```python
from build123d import *

# Parameters (mm, degrees)
F0_R      = 1.625
F1_DEPTH  = 8
F2_R      = 2.5
F2_R_2    = 1.625
F3_DEPTH  = 2
F4_R      = 3
F7_R      = 1.125
F8_DEPTH  = 16
F9_R      = 1.125
F10_DEPTH = 4.5
F11_R     = 1.125
F12_DEPTH = 6


with BuildPart() as f1:
    # F0 (on Right) → F1 (new body)
    with BuildSketch(Plane.YZ):
        with BuildLine():
            Line((0, -10), (0, 10))
            Line((0, 10), (-50, 10))
            ThreePointArc((-50, 10), (-60, 0), (-50, -10))
            Line((-50, -10), (0, -10))
        make_face()
        with Locations((-50, 0)):
            Circle(F0_R, mode=Mode.SUBTRACT)
    extrude(amount=F1_DEPTH)

    # F2 (on face) → F3 (join)
    with BuildSketch(Plane.YZ.offset(8)):
        with Locations((-50, 0)):
            Circle(F2_R)
        with Locations((-50, 0)):
            Circle(F2_R_2, mode=Mode.SUBTRACT)
    extrude(amount=F3_DEPTH)

    # F4
    f4_edges = [f1.edges().sort_by_distance(p)[0] for p in [
        (8, -25, 10),
    ]]
    fillet(f4_edges, radius=F4_R)

    # F5: F1 across plane


with BuildPart() as f1_1:
    add(f1.part)
    add(f1.part.mirror(Plane.YZ))

    # F6: F1 across plane


with BuildPart() as f1_2:
    add(f1_1.part)
    add(f1_1.part.mirror(Plane.XZ))

    # F7 (on face) → F8 (cut, through all)
    with BuildSketch(Plane.YZ.offset(8)):
        Polygon((15.6563942954, -6.5), (38.6563942954, -6.5), (38.6563942954, -2.5), (40.1563942954, -2.5), (40.1563942954, 2.5), (38.6563942954, 2.5), (38.6563942954, 6.5), (15.6563942954, 6.5), (15.6563942954, 2.5), (14.1563942954, 2.5), (14.1563942954, -2.5), (15.6563942954, -2.5), align=None)
        with Locations((12.6563942954, 0)):
            Circle(F7_R)
        with Locations((41.6563942954, 0)):
            Circle(F7_R)
    extrude(amount=-F8_DEPTH, mode=Mode.SUBTRACT)

    # F9 (on face) → F10 (cut)
    with BuildSketch(Plane.YZ.offset(8)):
        Polygon((15.6563942954, 6.5), (10.6563942954, 6.5), (10.6563942954, -6.5), (15.6563942954, -6.5), (15.6563942954, -2.5), (14.1563942954, -2.5), (14.1563942954, 2.5), (15.6563942954, 2.5), align=None)
        with Locations((12.6563942954, 0)):
            Circle(F9_R, mode=Mode.SUBTRACT)
        Polygon((43.6563942954, 6.5), (38.6563942954, 6.5), (38.6563942954, 2.5), (40.1563942954, 2.5), (40.1563942954, -2.5), (38.6563942954, -2.5), (38.6563942954, -6.5), (43.6563942954, -6.5), align=None)
        with Locations((41.6563942954, 0)):
            Circle(F9_R, mode=Mode.SUBTRACT)
    extrude(amount=-F10_DEPTH, mode=Mode.SUBTRACT)

    # F11 (on face) → F12 (cut)
    with BuildSketch(Plane(origin=(-8, 0, 0), x_dir=(0, -1, 0), z_dir=(-1, 0, 0))):
        Polygon((-43.6563942954, 6.5), (-43.6563942954, -6.5), (-38.6563942954, -6.5), (-38.6563942954, -2.5), (-40.1563942954, -2.5), (-40.1563942954, 2.5), (-38.6563942954, 2.5), (-38.6563942954, 6.5), align=None)
        with Locations((-41.6563942954, 0)):
            Circle(F11_R, mode=Mode.SUBTRACT)
        Polygon((-15.6563942954, -2.5), (-15.6563942954, -6.5), (-10.6563942954, -6.5), (-10.6563942954, 6.5), (-15.6563942954, 6.5), (-15.6563942954, 2.5), (-14.1563942954, 2.5), (-14.1563942954, -2.5), align=None)
        with Locations((-12.6563942954, 0)):
            Circle(F11_R, mode=Mode.SUBTRACT)
    extrude(amount=-F12_DEPTH, mode=Mode.SUBTRACT)


solid = f1_2.part
```
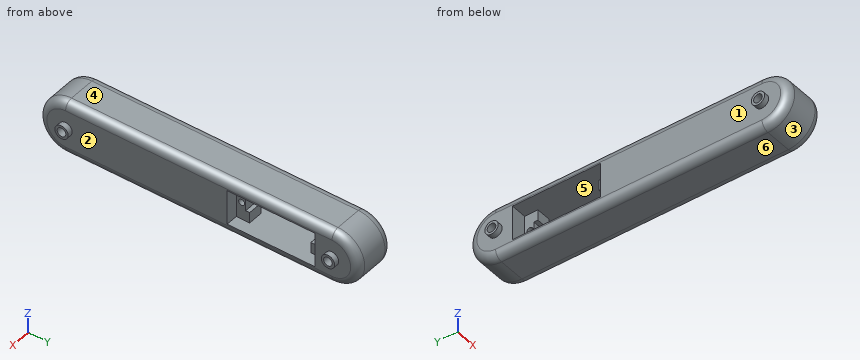
Work out the finished part from the listing and answer in its coordinate system (mm). Face numbers are marked on the shaded views. A direction names the side the tool comes from. Coordinates: 2 decimals unless noted, no trailing zeros. Order: outer loops, then holes, each group sorted by start corner. A loop starts at its lowest first (then second) coordinate and runs counter-clockwise, first axis right, second up. Notation, with made-up numbers: M 15.25,-16.5 L 68.25,-16.5 A19 ccw 68.25,20.5 Z; hole C 47,87 d11. An arc over 180 degrees is marked long. Use CSV: the item, a comma, the result in double quotes.
1) Section D-D on z = 0 is taken. Count the separate pieces of the cut face and the enclosed holes in it, plus the area to 3 significant figures.
Worked out:
separate pieces,"6"
enclosed holes,"0"
area,"1,310 mm^2"
2) Determine the mould class of the marked faces 4, 5 and 6 for opening direction Z: released by +Z, released by -Z, zero draft, split by the parting line, or undercut.
Worked out:
face 4,"released by +Z"
face 5,"undercut"
face 6,"released by -Z"
3) Section C-C on y = -31.5 is taken. Write down the section's boundary in (x, z).
Worked out:
outline,"M -8,-7 A3 ccw -5,-10 L 5,-10 A3 ccw 8,-7 L 8,7 A3 ccw 5,10 L -5,10 A3 ccw -8,7 Z"
4) Flat-ended cylindrical pins translate along their axes: pin 1 Ø2 at (x, z) = (4, 7) entering from +Y; pin 2 Ø3 at (y, z) = (-41.5, 7.5) entering from +X; pin 3 Ø1.5 at (y, z) = (41.5, 3) entering from +X; pin 4 Ø1.8 at (y, z) = (41.66, 0) entering from +X. Find the tip coordinate at first contact, or state that the pin passes through.
Worked out:
pin 1,"stops at y = 58"
pin 2,"stops at x = 8"
pin 3,"stops at x = 3.5"
pin 4,"passes through"
5) Section B-B on x = -3.5 is taken. Write down the section's boundary in (y, z) (3 decimals), plus the area to 3 significant figures.
Worked out:
outline,"M -50,-10 L 50,-10 A10 ccw 50,10 L -50,10 A10 ccw Z; hole C -50,0 d3.25; hole M 10.656,-6.5 L 43.656,-6.5 L 43.656,6.5 L 10.656,6.5 Z; hole C 50,0 d3.25"
area,"1,870 mm^2"
6) For the marked faces 1, 2 and 3, determine the directions among +Z, -Z, +X, -X, +Y, -Y from which every point of the face is accessible in a straight line to the end or side of a thin tool.
Worked out:
face 1,"-X"
face 2,"+X"
face 3,"+X, -X, -Y"
7) Section A-A on x = 1.5 is taken. Write down the section's boundary in (y, z) (3 decimals).
Worked out:
outline,"M -50,-10 L 50,-10 A10 ccw 50,10 L -50,10 A10 ccw Z; hole C -50,0 d3.25; hole C 12.656,0 d2.25; hole M 14.156,-2.5 L 15.656,-2.5 L 15.656,-6.5 L 38.656,-6.5 L 38.656,-2.5 L 40.156,-2.5 L 40.156,2.5 L 38.656,2.5 L 38.656,6.5 L 15.656,6.5 L 15.656,2.5 L 14.156,2.5 Z; hole C 41.656,0 d2.25; hole C 50,0 d3.25"
8) Consider line 1 (Z direction, x = -4.25, y = -50) (3 decimals); line 2 (Y direction, x = 1.5, z = 0.25); line 3 (Y direction, x = 7, z = -0.5). Determine where each line is inside the solid, lowest interval first. Write a range as [from, to].
Worked out:
line 1,"z = [-10, -1.625], [1.625, 10]"
line 2,"y = [-60, -51.61], [-48.39, 11.56], [13.75, 14.16], [40.16, 40.56], [42.75, 48.39], [51.61, 60]"
line 3,"y = [-59.22, -51.55], [-48.45, 10.66], [43.66, 48.45], [51.55, 59.22]"
